For this review, take the finished solid that the model builds, in its own axes (mm). Face numbers are marked on the shaded views. Coordinates: 2 decimals unless noted, no trailing zeros. Write each loop counter-clockwise with the first axis right and the second up, starting at its lowest first coordinate (ties: lowest second). Pieces come first, ordered by that corner, then holes. Notation, with made-up numbers: M 87,-33.75 L 100,-33.75 A11 cw 100,-22.75 Z; hole C -2.75,9.25 d4. An arc over 180 degrees is marked long. Return JSON: item names as keys, results as strings.
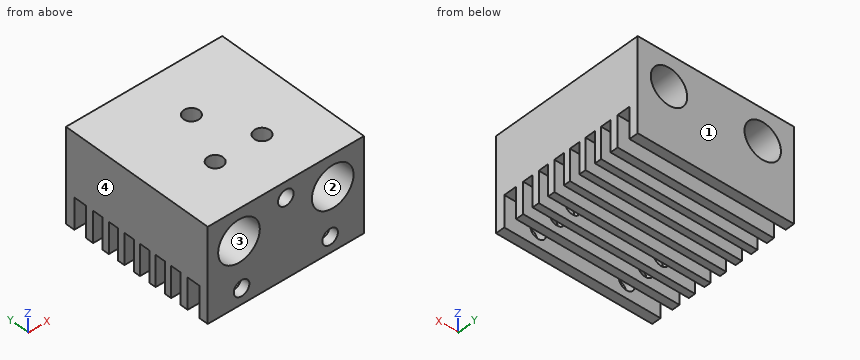
Autodesk Inventor part; units mm, degrees
ref_plane "YZ Plane" through (0, 0, 0) normal (1, 0, 0) x (0, 1, 0)
ref_plane "XZ Plane" through (0, 0, 0) normal (0, 1, 0) x (-1, 0, 0)
ref_plane "XY Plane" through (0, 0, 0) normal (0, 0, 1) x (1, 0, 0)
sketch "Sketch2" plane through (0, 0, 0) normal (0, 1, 0) x (-1, 0, 0)
  line L0 (-8, 10) -> (22, 10)
  line L1 (22, 10) -> (22, -8)
  line L2 (22, -8) -> (-8, -8)
  line L3 (-8, -8) -> (-8, 10)
  point P0 (0, 0)
  point P1 (-2, 4)
  point P2 (16, 4)
  point P3 (7, 7)
  point P4 (15.5, -5)
  point P5 (-1.5, -5)
  dimension "d0" = 30
  dimension "d1" = 18
  dimension "d2" = 6
  dimension "d3" = 6
  dimension "d4" = 6
  dimension "d5" = 6
  dimension "d40" = 15
  dimension "d41" = 3
  dimension "d42" = 6.5
  dimension "d43" = 6.5
  dimension "d44" = 3
  dimension "d45" = 3
extrude "Extrusion1" add sketch "Sketch2" along normal blind 30
hole "Hole1" at (2, 0, 4) at (-16, 0, 4) direction (0, 1, 0) diameter 7 end through all
hole "Hole2" at (-16, 0, 4) at (2, 0, 4) direction (0, 1, 0) diameter 8 depth 6.5 tip angle 118
sketch "Sketch3" plane through (8, 0, 10) normal (1, 0, 0) x (0, 0, -1)
  line L0 (18, 1.75) -> (12, 1.75)
  line L1 (12, 1.75) -> (12, 4.25)
  line L2 (12, 4.25) -> (18, 4.25)
  line L3 (18, 4.25) -> (18, 1.75)
  line L4 (18, 0) -> (0, 0)
  line L5 (18, 5.75) -> (12, 5.75)
  line L6 (12, 5.75) -> (12, 7.75)
  line L7 (12, 7.75) -> (18, 7.75)
  line L8 (18, 7.75) -> (18, 5.75)
  line L9 (18, 25.75) -> (12, 25.75)
  line L10 (12, 25.75) -> (12, 28.25)
  line L11 (12, 28.25) -> (18, 28.25)
  line L12 (18, 28.25) -> (18, 25.75)
  line L13 (18, 9.05) -> (12, 9.05)
  line L14 (12, 9.05) -> (12, 11.05)
  line L15 (12, 11.05) -> (18, 11.05)
  line L16 (18, 11.05) -> (18, 9.05)
  line L17 (18, 12.35) -> (12, 12.35)
  line L18 (12, 12.35) -> (12, 14.35)
  line L19 (12, 14.35) -> (18, 14.35)
  line L20 (18, 14.35) -> (18, 12.35)
  line L21 (18, 15.65) -> (12, 15.65)
  line L22 (12, 15.65) -> (12, 17.65)
  line L23 (12, 17.65) -> (18, 17.65)
  line L24 (18, 17.65) -> (18, 15.65)
  line L25 (18, 18.95) -> (12, 18.95)
  line L26 (12, 18.95) -> (12, 20.95)
  line L27 (12, 20.95) -> (18, 20.95)
  line L28 (18, 20.95) -> (18, 18.95)
  line L29 (18, 22.25) -> (12, 22.25)
  line L30 (12, 22.25) -> (12, 24.25)
  line L31 (12, 24.25) -> (18, 24.25)
  line L32 (18, 24.25) -> (18, 22.25)
  line L33 (0, 30) -> (18, 30)
  point P0 (10, 0)
  dimension "d22" = 6
  dimension "d23" = 2.5
  dimension "d24" = 1.75
  dimension "d25" = 6
  dimension "d26" = 2
  dimension "d27" = 1.5
  dimension "d36" = 6
  dimension "d37" = 2.5
  dimension "d46" = 6
  dimension "d47" = 2
  dimension "d48" = 1.3
  dimension "d49" = 6
  dimension "d50" = 2
  dimension "d51" = 6
  dimension "d52" = 2
  dimension "d53" = 6
  dimension "d54" = 2
  dimension "d55" = 6
  dimension "d56" = 2
  dimension "d57" = 1.75
  dimension "d58" = 1.5
extrude "Extrusion3" cut sketch "Sketch3" against normal blind 30
hole "Hole3" at (-7, 0, 7) at (-15.5, 0, -5) at (1.5, 0, -5) direction (0, 1, 0) diameter 3 depth 10
thread "Thread1"
thread "Thread2"
thread "Thread3"
sketch "Sketch4" plane through (-22, 0, 10) normal (0, 0, 1) x (1, 0, 0)
  line L0 (30, 0) -> (30, 30)
  line L1 (0, 30) -> (30, 30)
  point P0 (22, 0)
  point P1 (19.5, 10)
  point P2 (10.5, 10)
  point P3 (15, 20)
  dimension "d74" = 10.5
  dimension "d75" = 15
  dimension "d76" = 19.5
  dimension "d77" = 20
  dimension "d78" = 10
hole "Hole4" at (-2.5, 10, 10) at (-11.5, 10, 10) at (-7, 20, 10) direction (0, 0, -1) diameter 3 depth 10
thread "Thread4"
thread "Thread5"
thread "Thread6"
properties part number "Chimera Heatsink" material "Aluminum 6061, Welded"
1. We need section C-C (z = -5). Give the number of separate pieces and of enclosed holes in the cut face, plus the area to 3 significant figures.
Checks:
{"separate pieces": "15", "enclosed holes": "0", "area": "363 mm2"}
2. Draft analysis for pull direction X (two halves, no side actions). For the marked faces 1, 2, 3 and 4, state which applies: +X half, -X half, draft (parallel to the pull), parting line (faces both ways), or undercut.
Checks:
{"face 1": "draft", "face 2": "undercut", "face 3": "undercut", "face 4": "-X half"}
3. Wall thickness on L1, parallel to X at y = 16.25, z = 4; L2, parallel to X at y = 1.1, z = -5; L3, parallel to Z at x = -15.5, y = 8.1: over which ranges is each line inside the solid? List them lowest first. Write a range as from..to.
Checks:
{"L1": "-22..-19.5, -12.5..-1.5, 5.5..8", "L2": "-22..-17, -14..0, 3..8", "L3": "-8..-6.5, -3.5..0.54, 7.46..10"}
4. Clearance check with flat-ended pins moving along their axes: pin 1 Ø0.6 at (x, y) = (-5, 20) entering from -Z; pin 2 Ø1 at (x, z) = (3, 6) entering from +Y; pin 3 Ø1.8 at (x, z) = (-7, 7) entering from -Y; pin 4 Ø1.5 at (x, y) = (-6.5, 20) entering from +Z. State where each tip first meets the part, or that it passes through.
Checks:
{"pin 1": "z = -2", "pin 2": "through", "pin 3": "y = 10", "pin 4": "z = 0"}
5. We need section A-A (z = 4). State the section outline as (x, y) points, plus the area to 3 significant figures.
Checks:
{"outline": "M -22,0 L -20,0 L -20,6.5 L -19.5,6.8 L -19.5,30 L -22,30 Z; M -12.5,6.8 L -12,6.5 L -12,0 L -2,0 L -2,6.5 L -1.5,6.8 L -1.5,8.88 A1.5 cw long -1.5,11.12 L -1.5,30 L -12.5,30 L -12.5,11.12 A1.5 cw long -12.5,8.88 Z; M 5.5,6.8 L 6,6.5 L 6,0 L 8,0 L 8,30 L 5.5,30 Z; hole C -7,20 d3", "area": "447 mm2"}
6. We need section B-B (y = 13.5). State the section outline as (x, z) points.
Checks:
{"outline": "M -22,-2 L 8,-2 L 8,10 L -22,10 Z; hole C -16,4 d7; hole C 2,4 d7"}
7. We need section D-D (y = 20). State the section outline as (x, z) points.
Checks:
{"outline": "M -22,-2 L 8,-2 L 8,10 L -5.5,10 L -5.5,0 L -8.5,0 L -8.5,10 L -22,10 Z; hole C -16,4 d7; hole C 2,4 d7"}
